from build123d import *

# Parameters (mm, degrees)
EXTRUDE_1_DEPTH     = 28
SKETCH_2_W          = 5
SKETCH_2_H          = 20
CUT_EXTRUDE_1_DEPTH = 5
SKETCH_3_R          = 1.5
CUT_EXTRUDE_2_DEPTH = 118.133742985


with BuildPart() as part:
    # 草圖1 → 填料-伸長1 (new body)
    with BuildSketch(Plane.XY):
        Polygon((-17.451364004, -6.196122823), (-17.451364004, -11.196122823), (-22.451364004, -11.196122823), (-22.451364004, 105.303877177), (-17.451364004, 105.303877177), (-17.451364004, 100.303877177), (-17.451364004, 95.303877177), (-17.451364004, -1.196122823), (16.048635996, -1.196122823), (16.048635996, -6.196122823), align=None)
    extrude(amount=EXTRUDE_1_DEPTH)

    # 草圖2 → 除料-伸長1 (cut)
    with BuildSketch(Plane(origin=(0, 0, 28), x_dir=(-1, 0, 0), z_dir=(0, 0, -1))):
        with Locations((19.951364004, 47.053877177)):
            Rectangle(SKETCH_2_W, SKETCH_2_H)
    extrude(amount=CUT_EXTRUDE_1_DEPTH, mode=Mode.SUBTRACT)

    # 草圖3 → 除料-伸長2 (cut, through all)
    with BuildSketch(Plane.XZ.offset(6.196122823)):
        with Locations((-2.451364004, 13)):
            Circle(SKETCH_3_R)
    extrude(amount=-CUT_EXTRUDE_2_DEPTH, mode=Mode.SUBTRACT)


solid = part.part
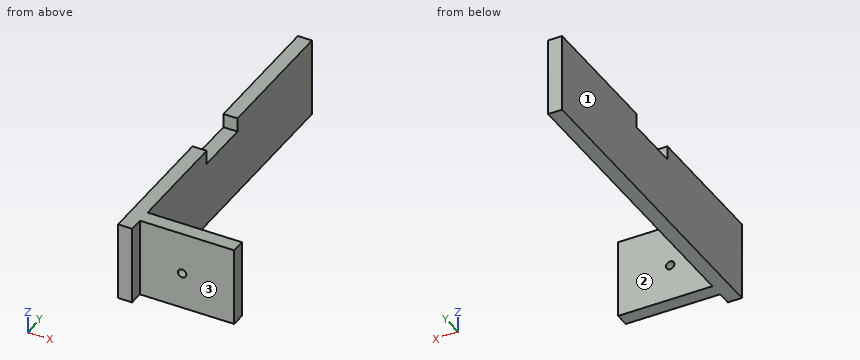
Model file for the job. Use its own axes, mm. Face numbers are marked on the shaded views. A direction names the side the tool comes from. Give positions to 0.01 mm unless a question says otherwise; leave off trailing zeros. Loops run counter-clockwise (first coordinate to the right, second up) from the corner with the lowest first, then second, coordinate; pieces in that order, holes last.
Item 1: Which spindle directions (+Z, -Z, +X, -X, +Y, -Y) get a long thin tool onto all of the face, cutting with end or side? Do the marked faces 1, 2 and 3. Say none if no direction does.
Check values:
face 1: +Z, -Z, -X, +Y, -Y
face 2: +Z, -Z, +X, +Y
face 3: +Z, -Z, +X, -Y
Item 2: Drop flat-ended pins along their axis: P1, Ø1.5, axis at x = 8.5, z = 23.5, coming from the -Y side; P2, Ø1, axis at y = 71, z = 7.5, coming from the +X side; P3, Ø8.5, axis at x = 5, z = 19.5, coming from the +Y side. Give the stop position or say it passes through.
Check values:
P1: stops at y = -6.2
P2: stops at x = -17.45
P3: stops at y = -1.2
Item 3: Slice it at C-C (z = 8.5). Write the cut outline in (x, y).
Check values:
outline: (-22.45, -11.2) - (-17.45, -11.2) - (-17.45, -6.2) - (16.05, -6.2) - (16.05, -1.2) - (-17.45, -1.2) - (-17.45, 105.3) - (-22.45, 105.3) - close
Item 4: Slice it at A-A (z = 25.25). Write the cut outline in (x, y).
Check values:
outline: (-22.45, -11.2) - (-17.45, -11.2) - (-17.45, -6.2) - (16.05, -6.2) - (16.05, -1.2) - (-17.45, -1.2) - (-17.45, 37.05) - (-22.45, 37.05) - close; (-22.45, 57.05) - (-17.45, 57.05) - (-17.45, 105.3) - (-22.45, 105.3) - close
Item 5: Drill centre lines: line 1 along Y through (x, z) = (5.5, 22.5); line 2 along X through (y, z) = (48.5, 1). Where is each one in solid material? Low to high.
Check values:
line 1: y = -6.2 to -1.2
line 2: x = -22.45 to -17.45
Item 6: Slice it at B-B (z = 13). Write the cut outline in (x, y).
Check values:
outline: (-22.45, -11.2) - (-17.45, -11.2) - (-17.45, -6.2) - (-3.95, -6.2) - (-3.95, -1.2) - (-17.45, -1.2) - (-17.45, 105.3) - (-22.45, 105.3) - close; (-0.95, -6.2) - (16.05, -6.2) - (16.05, -1.2) - (-0.95, -1.2) - close
Item 7: Slice it at D-D (x = -10). Write the cut outline in (y, z).
Check values:
outline: (-6.2, 0) - (-1.2, 0) - (-1.2, 28) - (-6.2, 28) - close
